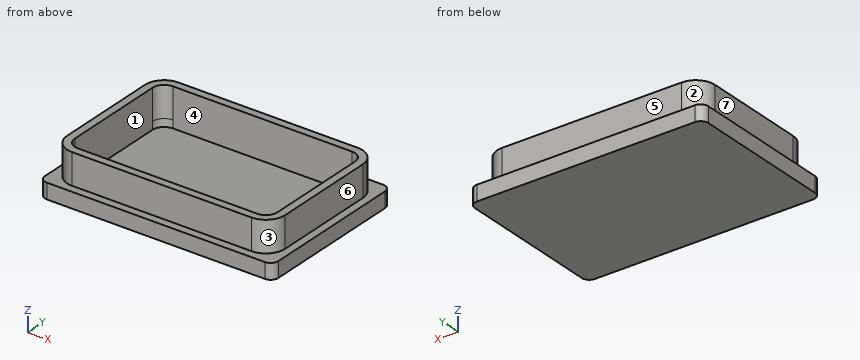
```python
from build123d import *

# Parameters (mm, degrees)
F1_DEPTH     = 5.08
F3_DEPTH     = 15.24
F4_T         = 2.54
F4_T3_DEPTH  = 64.008
F4_T5_DEPTH  = 39.243
F4_T8_ANGLE  = 90.000000001
F4_T10_ANGLE = 90.000000001
F4_T12_ANGLE = 90.000000001
F4_T14_ANGLE = 90.000000001


# Not quite as in the source:
# - a shell that OpenCascade refuses in one call is made with other operations: the cavity is built on its own and cut out
# - the program builds the solid bodies; features that only make, move or delete a surface that nothing else refers to are left out


with BuildPart() as f1:
    # F0 (on Top) → F1 (new body)
    with BuildSketch(Plane.XY):
        with BuildLine():
            Line((35.814, 26.035), (-35.814, 26.035))
            ThreePointArc((-35.814, 26.035), (-37.6100512242, 25.2910512242), (-38.354, 23.495))
            Line((-38.354, 23.495), (-38.354, -23.495))
            ThreePointArc((-38.354, -23.495), (-37.6100512242, -25.2910512242), (-35.814, -26.035))
            Line((-35.814, -26.035), (35.814, -26.035))
            ThreePointArc((35.814, -26.035), (37.6100512242, -25.2910512242), (38.354, -23.495))
            Line((38.354, -23.495), (38.354, 23.495))
            ThreePointArc((38.354, 23.495), (37.6100512242, 25.2910512242), (35.814, 26.035))
        make_face()
        with BuildLine():
            ThreePointArc((-35.814, 17.0815), (-33.9541280605, 21.5716280605), (-29.464, 23.4315))
            Line((-29.464, 23.4315), (29.464, 23.4315))
            ThreePointArc((29.464, 23.4315), (33.9541280605, 21.5716280605), (35.814, 17.0815))
            Line((35.814, 17.0815), (35.814, -17.0815))
            ThreePointArc((35.814, -17.0815), (33.9541280605, -21.5716280605), (29.464, -23.4315))
            Line((29.464, -23.4315), (-29.464, -23.4315))
            ThreePointArc((-29.464, -23.4315), (-33.9541280605, -21.5716280605), (-35.814, -17.0815))
            Line((-35.814, -17.0815), (-35.814, 17.0815))
        make_face(mode=Mode.SUBTRACT)
    extrude(amount=F1_DEPTH)

    # F0 (on Top) → F3 (join)
    with BuildSketch(Plane.XY):
        with BuildLine():
            Line((29.464, 23.4315), (-29.464, 23.4315))
            ThreePointArc((-29.464, 23.4315), (-33.9541280605, 21.5716280605), (-35.814, 17.0815))
            Line((-35.814, 17.0815), (-35.814, -17.0815))
            ThreePointArc((-35.814, -17.0815), (-33.9541280605, -21.5716280605), (-29.464, -23.4315))
            Line((-29.464, -23.4315), (29.464, -23.4315))
            ThreePointArc((29.464, -23.4315), (33.9541280605, -21.5716280605), (35.814, -17.0815))
            Line((35.814, -17.0815), (35.814, 17.0815))
            ThreePointArc((35.814, 17.0815), (33.9541280605, 21.5716280605), (29.464, 23.4315))
        make_face()
    extrude(amount=F3_DEPTH)

    # F4: shell of thickness 2.54, made by hand


with BuildPart() as f4_core1:
    # F4_t2: copy of F1
    add(f1.part)

    # the walls: a layer under each face that stays
    f4_faces = [f4_core1.faces().sort_by_distance(p)[0] for p in [
        (0, 26.035, 2.54),
        (0, 0, 0),
        (-35.7970666667, -24.2993333333, 5.08),
        (38.354, 0, 2.54),
        (-38.354, 0, 2.54),
        (0, -26.035, 2.54),
        (-33.9541280605, 21.5716280605, 10.16),
        (0, 23.4315, 10.16),
        (33.9541280605, 21.5716280605, 10.16),
        (35.814, 0, 10.16),
        (33.9541280605, -21.5716280605, 10.16),
        (0, -23.4315, 10.16),
        (-33.9541280605, -21.5716280605, 10.16),
        (-35.814, 0, 10.16),
    ]]
    thicken(f4_faces, amount=-F4_T, mode=Mode.SUBTRACT)

    # F4_s4 → F4_t3 (cut)
    with BuildSketch(Plane.YZ.offset(-32.004)):
        Polygon((23.4569, 5.1054), (23.4315, 2.54), (20.8915, 2.54), (20.8915, 5.08), align=None)
        Polygon((-23.4569, 5.1054), (-23.4315, 2.54), (-20.8915, 2.54), (-20.8915, 5.08), align=None)
    extrude(amount=F4_T3_DEPTH, mode=Mode.SUBTRACT)

    # F4_s6 → F4_t5 (cut)
    with BuildSketch(Plane.XZ.offset(-19.6215)):
        Polygon((35.8394, 5.1054), (35.814, 2.54), (33.274, 2.54), (33.274, 5.08), align=None)
        Polygon((-35.8394, 5.1054), (-35.814, 2.54), (-33.274, 2.54), (-33.274, 5.08), align=None)
    extrude(amount=F4_T5_DEPTH, mode=Mode.SUBTRACT)

    # F4_s7 → F4_t8 (revolve, cut)
    with BuildSketch(Plane.XZ.offset(-17.0815)):
        Polygon((-35.8394, 5.1054), (-35.814, 2.54), (-33.274, 2.54), (-33.274, 5.08), align=None)
    revolve(axis=Axis((-29.464, 17.0815, 5.08), (0, 0, -1)), revolution_arc=F4_T8_ANGLE, mode=Mode.SUBTRACT)

    # F4_s9 → F4_t10 (revolve, cut)
    with BuildSketch(Plane.YZ.offset(29.464)):
        Polygon((23.4569, 5.1054), (23.4315, 2.54), (20.8915, 2.54), (20.8915, 5.08), align=None)
    revolve(axis=Axis((29.464, 17.0815, 5.08), (0, 0, -1)), revolution_arc=F4_T10_ANGLE, mode=Mode.SUBTRACT)

    # F4_s11 → F4_t12 (revolve, cut)
    with BuildSketch(Plane.XZ.offset(17.0815)):
        Polygon((35.8394, 5.1054), (35.814, 2.54), (33.274, 2.54), (33.274, 5.08), align=None)
    revolve(axis=Axis((29.464, -17.0815, 5.08), (0, 0, -1)), revolution_arc=F4_T12_ANGLE, mode=Mode.SUBTRACT)

    # F4_s13 → F4_t14 (revolve, cut)
    with BuildSketch(Plane.YZ.offset(-29.464)):
        Polygon((-23.4569, 5.1054), (-23.4315, 2.54), (-20.8915, 2.54), (-20.8915, 5.08), align=None)
    revolve(axis=Axis((-29.464, -17.0815, 5.08), (0, 0, -1)), revolution_arc=F4_T14_ANGLE, mode=Mode.SUBTRACT)


with BuildPart() as f1_1:
    add(f1.part)

    # what is left inside the walls is the cavity
    f4_cavity = [f4_core1.part.solids().sort_by_distance(p)[0] for p in [
        (0, -6.963833, 2.5654),
    ]]
    add(f4_cavity, mode=Mode.SUBTRACT)


solid = f1_1.part
```
Verification items for the finished model (mm, model axes). Face numbers are marked on the shaded views. A direction names the side the tool comes from. Coordinates: 2 decimals unless noted, no trailing zeros. Write each loop counter-clockwise with the first axis right and the second up, starting at its lowest first coordinate (ties: lowest second). Pieces come first, ordered by that corner, then holes. Notation, with made-up numbers: (-31.5, 22.25) - (14.5, 22.25) arc R17 cw to (14.5, 35.25) - close; hole circle Ø11 at (10.5, 54). An arc over 180 degrees is marked (long way). One line per question, with ' | ' between items. Start each with the question number.
1. Section check D-D (y = 22). Enter the section's corners in (x, z).
2. Section check C-C (x = -15). Enter the section's corners in (y, z) (1 decimal).
3. Gauge pin test, flat ends, axial feed: P1, Ø21, axis at x = 0, y = -5, coming from the +Z side; P2, Ø3, axis at x = 10, z = 12, coming from the -Y side; P3, Ø1, axis at y = -17.5, z = 8.5, coming from the +X side. Record the tip position at first contact, or that the pin passes through.
4. Section check A-A (z = 13.25). Enter the section's corners in (x, y).
5. Draft check along X on the marked faces 1, 2 and 3. Enter one of: released by +X, released by -X, zero draft, split by the parting line, or undercut.
6. Access from +Z, -Z, +X, -X, +Y, -Y to the whole of each face (thin tool, end or side, straight path). Record for the marked faces 4, 5, 6 and 7.
7. Material ranges on line 1 along Y through (x, z) = (-9, 13.75); line 2 along X through (y, z) = (-3.5, 3.75); line 3 along X through (y, z) = (-11, 9.75), recorded low to high.
8. Section check B-B (y = -15). Enter the section's corners in (x, z), plus the area to 3 significant figures.
Computed values:
1) outline: (-38.35, 0) - (38.35, 0) - (38.35, 5.08) - (33.48, 5.08) - (33.48, 15.24) - (-33.48, 15.24) - (-33.48, 5.08) - (-38.35, 5.08) - close
2) outline: (-26, 0) - (26, 0) - (26, 5.1) - (23.4, 5.1) - (23.4, 15.2) - (20.9, 15.2) - (20.9, 2.5) - (-20.9, 2.5) - (-20.9, 15.2) - (-23.4, 15.2) - (-23.4, 5.1) - (-26, 5.1) - close
3) P1: z = 2.54 | P2: y = -23.43 | P3: x = 35.81
4) outline: (-35.81, -17.08) arc R6.35 ccw to (-29.46, -23.43) - (29.46, -23.43) arc R6.35 ccw to (35.81, -17.08) - (35.81, 17.08) arc R6.35 ccw to (29.46, 23.43) - (-29.46, 23.43) arc R6.35 ccw to (-35.81, 17.08) - close; hole (-33.27, -17.08) arc R3.81 ccw to (-29.46, -20.89) - (29.46, -20.89) arc R3.81 ccw to (33.27, -17.08) - (33.27, 17.08) arc R3.81 ccw to (29.46, 20.89) - (-29.46, 20.89) arc R3.81 ccw to (-33.27, 17.08) - close
5) face 1: undercut | face 2: released by -X | face 3: released by +X
6) face 4: +Z | face 5: +Z, +X, -X, +Y | face 6: +Z, +X, +Y, -Y | face 7: +Z, -X, +Y, -Y
7) line 1: -23.43 to -20.89, 20.89 to 23.43 | line 2: -38.35 to -33.27, 33.27 to 38.35 | line 3: -35.81 to -33.27, 33.27 to 35.81
8) outline: (-38.35, 0) - (38.35, 0) - (38.35, 5.08) - (35.81, 5.08) - (35.81, 15.24) - (33.27, 15.24) - (33.27, 2.54) - (-33.27, 2.54) - (-33.27, 15.24) - (-35.81, 15.24) - (-35.81, 5.08) - (-38.35, 5.08) - close | area: 272 mm²
